Part model, mm, in its own coordinate system. A direction names the side the tool comes from. Give positions to 0.01 mm unless a question says otherwise; leave off trailing zeros. Order: outer loops, then holes, each group sorted by start corner. A loop starts at its lowest first (then second) coordinate and runs counter-clockwise, first axis right, second up. Notation, with made-up numbers: (55, 87.25) - (67, 87.25) arc R14 ccw to (67, 114.25) - close; hole circle Ø4 at (-15, 6.25). An arc over 180 degrees is marked (long way). One line per item, written item: value.
```python
from build123d import *

# Parameters (mm, degrees)
ESQUISSE1_R      = 1.25
EXTRUSION1_DEPTH = 2
ESQUISSE2_R      = 3.548892627
ESQUISSE2_R_2    = 0.619205298
EXTRUSION2_DEPTH = 7
ESQUISSE3_W      = 9
ESQUISSE3_H      = 12
EXTRUSION3_DEPTH = 5


with BuildPart() as part:
    # Esquisse1 → Extrusion1 (new body)
    with BuildSketch(Plane(origin=(0, 0, 0), x_dir=(1, 0, 0), z_dir=(0, 1, 0))):
        with BuildLine():
            Line((-4.5, 6), (-4.5, -6))
            ThreePointArc((-4.5, -6), (0, -10.5), (4.5, -6))
            Line((4.5, -6), (4.5, 6))
            ThreePointArc((4.5, 6), (0, 10.5), (-4.5, 6))
        make_face()
        with Locations(Location((0, 7.5, 0), (0, 0, 270))):
            Circle(ESQUISSE1_R, mode=Mode.SUBTRACT)
        with Locations(Location((0, -7.5, 0), (0, 0, 270))):
            Circle(ESQUISSE1_R, mode=Mode.SUBTRACT)
    extrude(amount=-EXTRUSION1_DEPTH)

    # Esquisse2 → Extrusion2 (add)
    # profile 1 of 2: a face of its own
    with BuildSketch(Plane(origin=(0, 0, 0), x_dir=(-1, 0, 0), z_dir=(0, 1, 0))):
        with BuildLine():
            Line((4.5, -1.5), (4.5, 6))
            Line((4.5, 6), (-4.5, 6))
            Line((-4.5, 6), (-4.5, -1.5))
            ThreePointArc((-4.5, -1.5), (0, -6), (4.5, -1.5))
        make_face()
        with Locations(Location((0, -1.5, 0), (0, 0, 90))):
            Circle(ESQUISSE2_R, mode=Mode.SUBTRACT)
    # profile 2 of 2: a face of its own
    with BuildSketch(Plane(origin=(0, 0, 0), x_dir=(-1, 0, 0), z_dir=(0, 1, 0))):
        with Locations(Location((0, -1.5, 0), (0, 0, 90))):
            Circle(ESQUISSE2_R_2)
    extrude(amount=EXTRUSION2_DEPTH)

    # Esquisse3 → Extrusion3 (add)
    with BuildSketch(Plane.XZ.offset(2)):
        Rectangle(ESQUISSE3_W, ESQUISSE3_H)
    extrude(amount=EXTRUSION3_DEPTH)


solid = part.part
```
1) Cut at D-D, the plane x = -3. Give the cut face in (y, z).
Outcome:
outline: (-7, -6) - (-2, -6) - (-2, -9.35) - (0, -9.35) - (0, -4.85) - (7, -4.85) - (7, -3.4) - (0, -3.4) - (0, 0.4) - (7, 0.4) - (7, 6) - (0, 6) - (0, 9.35) - (-2, 9.35) - (-2, 6) - (-7, 6) - close
2) Drill centre lines: line 1 along Z through (x, y) = (-0.5, 0.5); line 2 along Y through (x, z) = (-3.5, -5.75); line 3 along Y through (x, z) = (-3.75, 6.25). Where is each one in solid material? Low to high. Write a range as from..to.
Outcome:
line 1: z = -5.97..-5.01, -1.87..-1.13, 2.01..6
line 2: y = -7..0
line 3: y = -2..0
3) Cut at C-C, the plane y = -1.5. Give the cut face in (x, z).
Outcome:
outline: (-4.5, -6) arc R4.5 ccw to (4.5, -6) - (4.5, 6) arc R4.5 ccw to (-4.5, 6) - close; hole circle Ø2.5 at (0, -7.5); hole circle Ø2.5 at (0, 7.5)
4) Cut at A-A, the plane x = 0. Give the cut face in (y, z), then the cut area to 3 significant figures.
Outcome:
outline: (-7, -6) - (-2, -6) - (-2, -6.25) - (0, -6.25) - (0, -6) - (7, -6) - (7, -5.05) - (0, -5.05) - (0, -2.12) - (7, -2.12) - (7, -0.88) - (0, -0.88) - (0, 2.05) - (7, 2.05) - (7, 6) - (0, 6) - (0, 6.25) - (-2, 6.25) - (-2, 6) - (-7, 6) - close; (-2, -10.5) - (0, -10.5) - (0, -8.75) - (-2, -8.75) - close; (-2, 8.75) - (0, 8.75) - (0, 10.5) - (-2, 10.5) - close
area: 135 mm^2
5) Pin check, flat tips, straight feed: pin 1 (1.5 mm diameter, centred on x = 0, z = -7.5, fed in from +Y); pin 2 (2 mm diameter, centred on x = 1.5, z = -8.5, fed in from -Y); pin 3 (1.3 mm diameter, centred on x = 0.5, z = 8, fed in from +Y). Stop position of each tip, or through.
Outcome:
pin 1: passes through
pin 2: stops at y = -2
pin 3: stops at y = 0
6) Which spindle directions (+Z, -Z, +X, -X, +Y, -Y) get a long thin tool onto all of the face, cutting with end or side? Do faces 4 (the flat face through (0, -2, -9)), 5 (the flat face through (0, 3, 6)), 6 (the cylindrical face through (-0.38, 3.45, -1.99)). Say none if no direction does.
Outcome:
face 4: -Z, +X, -X, -Y
face 5: +Z, +X, -X, +Y
face 6: +Y
7) Cut at B-B, the plane z = -7.5. Give the cut face in (x, y), then the cut area to 3 significant figures.
Outcome:
outline: (-4.24, -2) - (-1.25, -2) - (-1.25, 0) - (-4.24, 0) - close; (1.25, -2) - (4.24, -2) - (4.24, 0) - (1.25, 0) - close
area: 12.0 mm^2
8) Mould opens along X. For faces 1 (the flat face through (-4.5, 0, 1)), 2 (the flat face through (0, -4, -6)), 3 (the flat face through (1, 0, -2)) say: released by +X, released by -X, zero draft, split by the parting line, or undercut.
Outcome:
face 1: released by -X
face 2: zero draft
face 3: undercut
